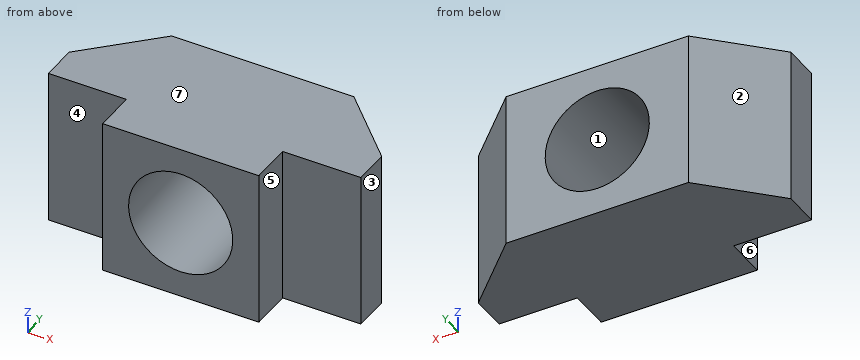
from build123d import *

# Parameters (mm, degrees)
EXTRUDE1_DEPTH     = 3
CUT_EXTRUDE1_REACH = 10.675
SKETCH2_R          = 2


with BuildPart() as part:
    # Sketch1 → Extrude1 (new, symmetric)
    with BuildSketch(Plane.XY):
        Polygon((-3, 0), (3, 0), (3, 1.6), (6, 1.6), (6, 3), (3.5, 5.5), (-3.5, 5.5), (-6, 3), (-6, 1.6), (-3, 1.6), align=None)
    extrude(amount=EXTRUDE1_DEPTH, both=True)

    # Sketch2 → Cut-Extrude1 (cut, up to next)
    with BuildSketch(Plane(origin=(0, 0, 0), x_dir=(1, 0, 0), z_dir=(0, 1, 0)), mode=Mode.PRIVATE) as cut_extrude1_sk1:
        with Locations(Location((0, 0, 0), (0, 0, 90))):
            Circle(SKETCH2_R)
    cut_extrude1_tool1 = extrude(cut_extrude1_sk1.sketch, amount=CUT_EXTRUDE1_REACH, mode=Mode.PRIVATE) & part.part
    add(cut_extrude1_tool1.solids().sort_by_distance((0, 0, 0))[0], mode=Mode.SUBTRACT)


solid = part.part
Here's how the part is built. I have some questions about the finished solid (model axes, mm). Face numbers are marked on the shaded views. A direction names the side the tool comes from. Give positions to 0.01 mm unless a question says otherwise; leave off trailing zeros. Order: outer loops, then holes, each group sorted by start corner. A loop starts at its lowest first (then second) coordinate and runs counter-clockwise, first axis right, second up. Notation, with made-up numbers: M -2,2 L 27,2 A10 ccw 27,14 Z; hole C 60,-13 d6. An arc over 180 degrees is marked long. Answer as a JSON object with one key per item and string values. Group by question number.
1) Suppose I cut it at D-D, the plane z = 2.25. Write out the boundary of the cut face in (x, y), plus the area to 4 significant figures.
2) Suppose I cut it at C-C, the plane x = 0. Write out the boundary of the cut face in (y, z), plus the area to 3 significant figures.
3) I'm going to push flat-ended pins straight in: pin 1 Ø2.5 at (x, z) = (4.5, 0) entering from -Y; pin 2 Ø1.8 at (y, z) = (0.5, -1) entering from +X. Where does each tip first touch, or does it pass through?
4) We'd pull the mould along X, two halves only. Please class the marked faces 1, 2, 3 and 4: pulls with the +X half, pulls with the -X half, needs draft (parallel to the pull), parting line crosses it, or undercut.
5) On a 3-axis mill with a long thin cutter (end or side, diameter ignored), from which of +Z, -Z, +X, -X, +Y, -Y can I reach the whole of each face in a straight line? I mean the marked faces 5, 6 and 7. Say none if no direction works.
6) Please list where these lines run through material, in increasing order: L1, parallel to X at y = 2.85, z = 0; L2, parallel to X at y = 0.5, z = 2.45; L3, parallel to X at y = 3.7, z = -0.85. Write a range as [from, to].
7) Suppose I cut it at A-A, the plane z = 0. Write out the boundary of the cut face in (x, y), plus the area to 4 significant figures.
8) Suppose I cut it at B-B, the plane y = 2.2. Write out the boundary of the cut face in (x, z), plus the area to 3 significant figures.
Results found:
{
 "1": {"outline": "M -6,1.6 L -3,1.6 L -3,0 L 3,0 L 3,1.6 L 6,1.6 L 6,3 L 3.5,5.5 L -3.5,5.5 L -6,3 Z", "area": "50.15 mm²"},
 "2": {"outline": "M 0,-3 L 5.5,-3 L 5.5,-2 L 0,-2 Z; M 0,2 L 5.5,2 L 5.5,3 L 0,3 Z", "area": "11.0 mm²"},
 "3": {"pin 1": "y = 1.6", "pin 2": "x = 3"},
 "4": {"face 1": "undercut", "face 2": "pulls with the -X half", "face 3": "pulls with the +X half", "face 4": "needs draft"},
 "5": {"face 5": "+Z, -Z, +X, -Y", "face 6": "+Z, -Z, -X, -Y", "face 7": "+Z, +X, -X, +Y, -Y"},
 "6": {"L1": "[-6, -2], [2, 6]", "L2": "[-3, 3]", "L3": "[-5.3, -1.81], [1.81, 5.3]"},
 "7": {"outline": "M -6,1.6 L -3,1.6 L -3,0 L -2,0 L -2,5.5 L -3.5,5.5 L -6,3 Z; M 2,0 L 3,0 L 3,1.6 L 6,1.6 L 6,3 L 3.5,5.5 L 2,5.5 Z", "area": "28.15 mm²"},
 "8": {"outline": "M -6,-3 L 6,-3 L 6,3 L -6,3 Z; hole C 0,0 d4", "area": "59.4 mm²"}
}
